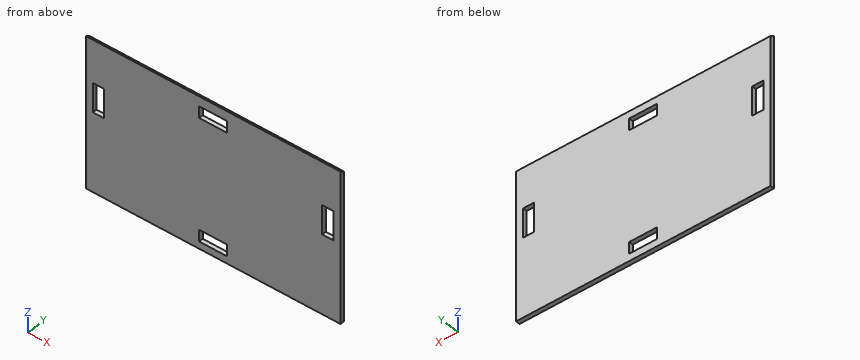
```python
from build123d import *

# Parameters (mm, degrees)
BOSS_EXTRUDE1_DEPTH = 181
SKETCH2_W           = 20
SKETCH2_H           = 8
SKETCH2_W_2         = 8
SKETCH2_H_2         = 20
CUT_EXTRUDE1_DEPTH  = 4
SKETCH3_W           = 11.684269825
SKETCH3_H           = 21.954659585
BOSS_EXTRUDE2_DEPTH = 3


with BuildPart() as part:
    # Sketch1 → Boss-Extrude1 (new body)
    with BuildSketch(Plane(origin=(0, 0, 0), x_dir=(0, 0, -1), z_dir=(1, 0, 0))):
        Polygon((0.351294643, 16.181618247), (2.08334545, 19.181618247), (104.351294643, 19.181618247), (104.351294643, 16.181618247), align=None)
    extrude(amount=-BOSS_EXTRUDE1_DEPTH)

    # Sketch2 → Cut-Extrude1 (cut)
    with BuildSketch(Plane(origin=(0, 19.181618247, 0), x_dir=(1, 0, 0), z_dir=(0, 1, 0))):
        with Locations((-90.499224225, 95.351294643)):
            Rectangle(SKETCH2_W, SKETCH2_H)
        with Locations((-8.999224225, 39.831548681)):
            Rectangle(SKETCH2_W_2, SKETCH2_H_2)
    cut_extrude1 = extrude(amount=-CUT_EXTRUDE1_DEPTH, mode=Mode.SUBTRACT)

    # Mirror1: Cut-Extrude1 across plane
    add(cut_extrude1.mirror(Plane.ZY.offset(90.499224225)), mode=Mode.SUBTRACT)

    # Mirror2: Cut-Extrude1 across plane
    add(cut_extrude1.mirror(Plane(origin=(0, 0, -53.216294643), x_dir=(1, 0, 0), z_dir=(0, 0, -1))), mode=Mode.SUBTRACT)

    # Sketch3 → Boss-Extrude2 (add)
    with BuildSketch(Plane(origin=(0, 19.181618247, 0), x_dir=(1, 0, 0), z_dir=(0, 1, 0))):
        with Locations((-10.841359137, 66.584328743)):
            Rectangle(SKETCH3_W, SKETCH3_H)
    extrude(amount=-BOSS_EXTRUDE2_DEPTH)


solid = part.part
```
Read the model definition and answer for the solid it produces. Units are mm, in the model's axes. Round coordinates to 2 decimals unless told otherwise and drop trailing zeros. Write each loop counter-clockwise with the first axis right and the second up, starting at its lowest first coordinate (ties: lowest second). Pieces come first, ordered by that corner, then holes. Notation, with made-up numbers: (71, 47.5) - (128, 47.5) arc R30 cw to (128, 83.5) - close; hole circle Ø3 at (72, -25). An arc over 180 degrees is marked (long way). One line per item, written item: value.
Q1. Find section B-B (z = -43). Determine the outline of the cut face in (x, y), and give its area (3 significant figures).
The answers:
outline: (-181, 16.18) - (-176, 16.18) - (-176, 19.18) - (-181, 19.18) - close; (-168, 16.18) - (-13, 16.18) - (-13, 19.18) - (-168, 19.18) - close; (-5, 16.18) - (0, 16.18) - (0, 19.18) - (-5, 19.18) - close
area: 495 mm2
Q2. Find section A-A (x = -11). Determine the outline of the cut face in (y, z).
The answers:
outline: (16.18, -104.35) - (19.18, -104.35) - (19.18, -49.83) - (16.18, -49.83) - close; (16.18, -29.83) - (19.18, -29.83) - (19.18, -2.08) - (16.18, -0.35) - close
Q3. This flat-tipped pin is pushed along its axis until it touches: P1, Ø1.5, axis at x = -89, y = 17.5, coming from the +Z side. Where does it stop, or does it pass through?
The answers:
P1: stops at z = -0.68
Q4. Find section D-D (y = 17.6). Determine the outline of the cut face in (x, z).
The answers:
outline: (-181, -104.35) - (0, -104.35) - (0, -1.17) - (-181, -1.17) - close; hole (-176, -49.83) - (-168, -49.83) - (-168, -29.83) - (-176, -29.83) - close; hole (-100.5, -99.35) - (-80.5, -99.35) - (-80.5, -91.35) - (-100.5, -91.35) - close; hole (-100.5, -15.08) - (-80.5, -15.08) - (-80.5, -7.08) - (-100.5, -7.08) - close; hole (-13, -49.83) - (-5, -49.83) - (-5, -29.83) - (-13, -29.83) - close
Q5. Straight lines are drawn through the part: line 1 (X direction, y = 16.95, z = -43); line 2 (Z direction, x = -91.5, y = 18); line 3 (Z direction, x = -79.5, y = 17). For each, find the intervals that lie inside material, in ascending order. Write a range as from..to.
The answers:
line 1: x = -181..-176, -168..-13, -5..0
line 2: z = -104.35..-99.35, -91.35..-15.08, -7.08..-1.4
line 3: z = -104.35..-0.82
Q6. Find section C-C (x = -85). Determine the outline of the cut face in (y, z).
The answers:
outline: (16.18, -104.35) - (19.18, -104.35) - (19.18, -99.35) - (16.18, -99.35) - close; (16.18, -91.35) - (19.18, -91.35) - (19.18, -15.08) - (16.18, -15.08) - close; (16.18, -7.08) - (19.18, -7.08) - (19.18, -2.08) - (16.18, -0.35) - close
